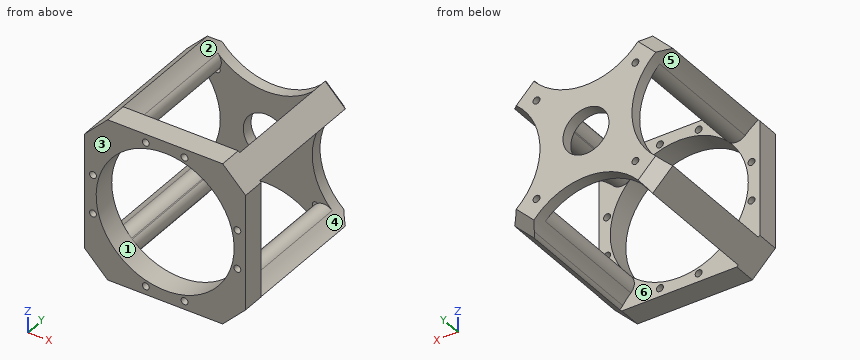
```python
from build123d import *

# Parameters (mm, degrees)
SKETCH1_W           = 70
SKETCH1_H           = 70
SKETCH1_R           = 30
SKETCH1_R_2         = 1.5
BOSS_EXTRUDE1_DEPTH = 65
SKETCH2_W           = 70
SKETCH2_H           = 70
SKETCH2_R           = 1.5
SKETCH2_R_2         = 10
BOSS_EXTRUDE2_DEPTH = 5
SKETCH3_R           = 30
CUT_EXTRUDE1_DEPTH  = 60
CIRPATTERN1_COUNT   = 4
FILLET2_R           = 5.1
CHAMFER1_SIZE       = 10
CHAMFER2_SIZE       = 5


with BuildPart() as part:
    # Sketch1 → Boss-Extrude1 (new body)
    with BuildSketch(Plane(origin=(0, 0, 0), x_dir=(1, 0, 0), z_dir=(0, 1, 0))):
        Rectangle(SKETCH1_W, SKETCH1_H)
        with Locations(Location((0, 0, 0), (0, 0, 270))):
            Circle(SKETCH1_R, mode=Mode.SUBTRACT)
        with Locations(Location((-8.411618966, 31.392589354, 0), (0, 0, 270))):
            Circle(SKETCH1_R_2, mode=Mode.SUBTRACT)
        with Locations(Location((8.411618966, 31.392589354, 0), (0, 0, 270))):
            Circle(SKETCH1_R_2, mode=Mode.SUBTRACT)
        with Locations(Location((31.392589354, 8.411618966, 0), (0, 0, 270))):
            Circle(SKETCH1_R_2, mode=Mode.SUBTRACT)
        with Locations(Location((31.392589354, -8.411618966, 0), (0, 0, 270))):
            Circle(SKETCH1_R_2, mode=Mode.SUBTRACT)
        with Locations(Location((8.411618966, -31.392589354, 0), (0, 0, 270))):
            Circle(SKETCH1_R_2, mode=Mode.SUBTRACT)
        with Locations(Location((-8.411618966, -31.392589354, 0), (0, 0, 270))):
            Circle(SKETCH1_R_2, mode=Mode.SUBTRACT)
        with Locations(Location((-31.392589354, -8.411618966, 0), (0, 0, 270))):
            Circle(SKETCH1_R_2, mode=Mode.SUBTRACT)
        with Locations(Location((-31.392589354, 8.411618966, 0), (0, 0, 270))):
            Circle(SKETCH1_R_2, mode=Mode.SUBTRACT)
    extrude(amount=BOSS_EXTRUDE1_DEPTH)

    # Sketch2 → Boss-Extrude2 (add)
    with BuildSketch(Plane(origin=(0, 65, 0), x_dir=(1, 0, 0), z_dir=(0, 1, 0))):
        Rectangle(SKETCH2_W, SKETCH2_H)
        with Locations(Location((0, 32.5, 0), (0, 0, 270))):
            Circle(SKETCH2_R, mode=Mode.SUBTRACT)
        with Locations(Location((16.25, 28.145825623, 0), (0, 0, 270))):
            Circle(SKETCH2_R, mode=Mode.SUBTRACT)
        with Locations(Location((28.145825623, 16.25, 0), (0, 0, 270))):
            Circle(SKETCH2_R, mode=Mode.SUBTRACT)
        with Locations(Location((32.5, 0, 0), (0, 0, 270))):
            Circle(SKETCH2_R, mode=Mode.SUBTRACT)
        with Locations(Location((28.145825623, -16.25, 0), (0, 0, 270))):
            Circle(SKETCH2_R, mode=Mode.SUBTRACT)
        with Locations(Location((16.25, -28.145825623, 0), (0, 0, 270))):
            Circle(SKETCH2_R, mode=Mode.SUBTRACT)
        with Locations(Location((0, -32.5, 0), (0, 0, 270))):
            Circle(SKETCH2_R, mode=Mode.SUBTRACT)
        with Locations(Location((-16.25, -28.145825623, 0), (0, 0, 270))):
            Circle(SKETCH2_R, mode=Mode.SUBTRACT)
        with Locations(Location((-28.145825623, -16.25, 0), (0, 0, 270))):
            Circle(SKETCH2_R, mode=Mode.SUBTRACT)
        with Locations(Location((-32.5, 0, 0), (0, 0, 270))):
            Circle(SKETCH2_R, mode=Mode.SUBTRACT)
        with Locations(Location((-28.145825623, 16.25, 0), (0, 0, 270))):
            Circle(SKETCH2_R, mode=Mode.SUBTRACT)
        with Locations(Location((-16.25, 28.145825623, 0), (0, 0, 270))):
            Circle(SKETCH2_R, mode=Mode.SUBTRACT)
        with Locations(Location((0, 0, 0), (0, 0, 270))):
            Circle(SKETCH2_R_2, mode=Mode.SUBTRACT)
        with Locations(Location((-21.5, 21.5, 0), (0, 0, 27.946923368))):
            Circle(SKETCH2_R, mode=Mode.SUBTRACT)
        with Locations(Location((21.5, 21.5, 0), (0, 0, 152.053076632))):
            Circle(SKETCH2_R, mode=Mode.SUBTRACT)
        with Locations(Location((21.5, -21.5, 0), (0, 0, 62.053076632))):
            Circle(SKETCH2_R, mode=Mode.SUBTRACT)
        with Locations(Location((-21.5, -21.5, 0), (0, 0, 117.946923368))):
            Circle(SKETCH2_R, mode=Mode.SUBTRACT)
    extrude(amount=BOSS_EXTRUDE2_DEPTH)

    # Sketch3 → Cut-Extrude1 (cut)
    with BuildSketch(Plane(origin=(0, 70, 0), x_dir=(1, 0, 0), z_dir=(0, 1, 0))):
        with Locations((0, 50)):
            Circle(SKETCH3_R)
    cut_extrude1 = extrude(amount=-CUT_EXTRUDE1_DEPTH, mode=Mode.SUBTRACT)

    # CirPattern1: Cut-Extrude1 ×4 about axis
    cirpattern1_axis = Axis((0, 0, 0), (0, 1, 0))
    for i in range(1, CIRPATTERN1_COUNT):
        add(cut_extrude1.rotate(cirpattern1_axis, i * 360 / CIRPATTERN1_COUNT), mode=Mode.SUBTRACT)

    # Fillet2
    # the kernel refuses this fillet: 5.1 mm, written as the material it takes off along each edge
    with BuildSketch(Plane(origin=(25.980762114, 10, -35), x_dir=(1, 0, 0), z_dir=(0, 1, 0))) as fillet2_piece_1:
        with BuildLine():
            CenterArc((2.794227026, -5.1), FILLET2_R, 90, 55.064804049)
            ThreePointArc((-1.386754302, -2.179487179), (-0.669907143, -1.104676981), (0, 0))
            Line((0, 0), (2.794227026, 0))
        make_face()
    extrude(amount=66.985567566, mode=Mode.SUBTRACT)
    with BuildSketch(Plane(origin=(16.583123952, 65, -25), x_dir=(0.7763821649146441, 0, 0.6302624326440933), z_dir=(0, -1, 0)), Plane(origin=(16.583123952, 65, 25), x_dir=(0.776382164914642, 0, 0.6302624326440961), z_dir=(0, -1, 0)), Plane(origin=(25, 65, 16.583123952), x_dir=(-0.6302624326440963, 0, 0.7763821649146417), z_dir=(0, -1, 0)), Plane(origin=(-25, 65, 16.583123952), x_dir=(-0.630262432644093, 0, 0.7763821649146444), z_dir=(0, -1, 0))) as fillet2_piece_2:
        with BuildLine():
            CenterArc((6.253330537, -5.076416608), FILLET2_R, 95.512177233, 90.836671542)
            ThreePointArc((1.184608644, -5.640383249), (0.728068224, -2.79167812), (0, 0))
            ThreePointArc((0, 0), (2.881719141, -0.138725834), (5.763438283, 0))
        make_face()
    extrude(amount=55, mode=Mode.SUBTRACT)
    with BuildSketch(Plane(origin=(-16.583123952, 65, -25), x_dir=(-0.7763821649146441, 0, 0.6302624326440932), z_dir=(0, -1, 0)), Plane(origin=(-16.583123952, 65, 25), x_dir=(-0.7763821649146462, 0, 0.6302624326440908), z_dir=(0, -1, 0)), Plane(origin=(25, 65, -16.583123952), x_dir=(-0.6302624326440941, 0, -0.7763821649146434), z_dir=(0, -1, 0)), Plane(origin=(-25, 65, -16.583123952), x_dir=(-0.6302624326440903, 0, -0.7763821649146465), z_dir=(0, -1, 0))) as fillet2_piece_3:
        with BuildLine():
            CenterArc((6.253330537, 5.076416608), FILLET2_R, 173.651151224, 90.836671542)
            ThreePointArc((1.184608644, 5.640383249), (0.728068224, 2.79167812), (0, 0))
            ThreePointArc((0, 0), (2.881719141, 0.138725834), (5.763438283, 0))
        make_face()
    extrude(amount=55, mode=Mode.SUBTRACT)

    # Chamfer1
    # the kernel refuses this chamfer: 10 mm, written as the material it takes off along each edge
    with BuildSketch(Plane(origin=(35, -25.71682988, 35), x_dir=(-0.9996219169112968, 0, 0.027495876610586317), z_dir=(0, 1, 0)), Plane(origin=(-35, 95.71682988, 35), x_dir=(0.9996219169112968, 0, 0.027495876610586317), z_dir=(0, -1, 0))) as chamfer1_piece_1:
        Polygon((CHAMFER1_SIZE * 0.999621916911, -CHAMFER1_SIZE * 0.0274958766106), (-CHAMFER1_SIZE * 0.0274958766106, -CHAMFER1_SIZE * 0.999621916911), (0, 0), align=None)
    extrude(amount=121.433659759, mode=Mode.SUBTRACT)
    with BuildSketch(Plane(origin=(35, -25.71682988, -35), x_dir=(-0.9996219169112968, 0, -0.027495876610586317), z_dir=(0, 1, 0)), Plane(origin=(-35, 95.71682988, -35), x_dir=(0.9996219169112968, 0, -0.027495876610586317), z_dir=(0, -1, 0))) as chamfer1_piece_2:
        Polygon((CHAMFER1_SIZE * 0.999621916911, CHAMFER1_SIZE * 0.0274958766106), (-CHAMFER1_SIZE * 0.0274958766106, CHAMFER1_SIZE * 0.999621916911), (0, 0), align=None)
    extrude(amount=121.433659759, mode=Mode.SUBTRACT)

    # Chamfer2
    chamfer2_edges = [part.edges().sort_by_distance(p)[0] for p in [
        (-30, 70, 30),
        (30, 70, 30),
        (30.138549403, 70, -29.861450597),
        (-30, 70, -30),
    ]]
    chamfer(chamfer2_edges, length=CHAMFER2_SIZE)


solid = part.part
```
Verification items for the finished model (mm, model axes). Face numbers are marked on the shaded views. A direction names the side the tool comes from. Round coordinates to 2 decimals unless told otherwise and drop trailing zeros. Order: outer loops, then holes, each group sorted by start corner. A loop starts at its lowest first (then second) coordinate and runs counter-clockwise, first axis right, second up.
1) Depth check by flat-ended pin: pin 1 (5 mm diameter, centred on x = -26, y = 36.5, fed in from +Z); pin 2 (17 mm diameter, centred on x = 6.5, z = 0, fed in from -Y); pin 3 (15 mm diameter, centred on x = -30.5, z = 3.5, fed in from +Y). Enter the tip coordinate at first touch or a pass-through.
Geometry says:
pin 1: stops at z = 34.38
pin 2: stops at y = 65
pin 3: stops at y = 10
2) Material ranges on line 1 (Y direction, x = -19, z = 24); line 2 (Y direction, x = -15, z = -19.5); line 3 (Z direction, x = -31, y = 41), recorded low to high.
Geometry says:
line 1: y = 0 to 10, 65 to 70
line 2: y = 65 to 70
line 3: z = -29 to -23.22, 23.22 to 29
3) Cross-section at B-B, the plane x = 0. Record the cut outline in (y, z).
Geometry says:
outline: (0, -35) - (10, -35) - (10, -30) - (0, -30) - close; (0, 30) - (10, 30) - (10, 35) - (0, 35) - close; (65, -20) - (70, -20) - (70, -10) - (65, -10) - close; (65, 10) - (70, 10) - (70, 20) - (65, 20) - close
4) Tool access check on the marked faces 1, 2 and 3. Record the directions out of +Z, -Z, +X, -X, +Y, -Y that give a thin tool (end or side, any length) a straight path to the whole face; none if there is none.
Geometry says:
face 1: -Y
face 2: +Z, +Y
face 3: +Z, -Z, +X, -X, -Y
5) Draft check along X on the marked faces 4, 5 and 6. Enter one of: +X half, -X half, draft (parallel to the pull), parting line (faces both ways), or undercut.
Geometry says:
face 4: +X half
face 5: -X half
face 6: undercut
6) Cross-section at A-A, the plane z = 0. Record the cut outline in (x, y).
Geometry says:
outline: (-35, 0) - (-30, 0) - (-30, 10) - (-35, 10) - close; (-20, 65) - (-10, 65) - (-10, 70) - (-20, 70) - close; (10, 65) - (20, 65) - (20, 70) - (10, 70) - close; (30, 0) - (35, 0) - (35, 10) - (30, 10) - close
7) Cross-section at D-D, the plane z = -12. Record the cut outline in (x, y).
Geometry says:
outline: (-35, 0) - (-27.5, 0) - (-27.5, 10) - (-35, 10) - close; (-22.5, 65) - (22.5, 65) - (22.5, 70) - (-22.5, 70) - close; (27.5, 0) - (35, 0) - (35, 10) - (27.5, 10) - close
8) Cross-section at C-C, the plane y = 23.5. Record the cut outline in (x, z), plus the area to 3 significant figures.
Geometry says:
outline: (-34.38, -25.62) - (-25.62, -34.38) arc R30 cw to (-21.06, -28.63) arc R5.1 ccw to (-21.06, -21.37) arc R30 cw to (-21.37, -21.06) arc R5.1 ccw to (-28.63, -21.06) arc R30 cw to start; (-34.38, 25.62) arc R30 cw to (-28.63, 21.06) arc R5.1 ccw to (-21.37, 21.06) arc R30 cw to (-21.06, 21.37) arc R5.1 ccw to (-21.06, 28.63) arc R30 cw to (-25.62, 34.38) - close; (21.06, -28.63) arc R30 cw to (24.59, -32.82) arc R5.1 ccw to (25.89, -34.11) - (34.38, -25.62) arc R30 cw to (28.63, -21.06) arc R5.1 ccw to (21.37, -21.06) arc R30 cw to (21.06, -21.37) arc R5.1 ccw to start; (21.06, 21.37) arc R30 cw to (21.37, 21.06) arc R5.1 ccw to (28.63, 21.06) arc R30 cw to (34.38, 25.62) - (25.62, 34.38) arc R30 cw to (21.06, 28.63) arc R5.1 ccw to start
area: 503 mm2
